```python
from build123d import *

# Parameters (mm, degrees)
BOSS_EXTRUDE1_DEPTH = 12.2
SKETCH2_R           = 1
CUT_EXTRUDE1_DEPTH  = 12.5
SKETCH3_R           = 2.5
BOSS_EXTRUDE2_DEPTH = 4
CUT_EXTRUDE2_DEPTH  = 7.5
SKETCH5_W           = 2.772136711
SKETCH5_H           = 1.05
SKETCH5_W_2         = 2.613565213
SKETCH5_H_2         = 1
CUT_EXTRUDE3_DEPTH  = 7.5


with BuildPart() as part:
    # Sketch1 → Boss-Extrude1 (new body)
    with BuildSketch(Plane.XY):
        Polygon((-5.25, 21), (-5.25, 18.3), (0, 18.3), (0, 0), (22.9, 0), (22.9, 18.3), (28.15, 18.3), (28.15, 21), (22.9, 21), (22.9, 28.5), (0, 28.5), (0, 21), align=None)
    extrude(amount=BOSS_EXTRUDE1_DEPTH)

    # Sketch2 → Cut-Extrude1 (cut)
    with BuildSketch(Plane(origin=(0, 21, 0), x_dir=(1, 0, 0), z_dir=(0, 1, 0))):
        with Locations((-2.55, -6.1)):
            Circle(SKETCH2_R)
        with Locations((25.45, -6.1)):
            Circle(SKETCH2_R)
    extrude(amount=-CUT_EXTRUDE1_DEPTH, mode=Mode.SUBTRACT)

    # Sketch3 → Boss-Extrude2 (add)
    with BuildSketch(Plane(origin=(0, 28.5, 0), x_dir=(1, 0, 0), z_dir=(0, 1, 0))):
        with Locations((6.05, -6.1)):
            Circle(SKETCH3_R)
    extrude(amount=BOSS_EXTRUDE2_DEPTH)

    # Sketch4 → Cut-Extrude2 (cut)
    with BuildSketch(Plane(origin=(0, 28.5, 0), x_dir=(1, 0, 0), z_dir=(0, 1, 0))):
        with BuildLine():
            Line((6.050000045, 0), (0, 0))
            Line((0, 0), (0, -5.320577137))
            ThreePointArc((0, -5.320577137), (2.021630587, -1.519362504), (6.050000045, 0))
        make_face()
        with BuildLine():
            Line((22.9, 0), (6.050000045, 0))
            ThreePointArc((6.050000045, 0), (9.58624096, -1.129587555), (11.812811814, -4.1))
            Line((11.812811814, -4.1), (15.4, -4.1))
            ThreePointArc((15.4, -4.1), (17.4, -6.1), (15.4, -8.1))
            Line((15.4, -8.1), (11.812811814, -8.1))
            ThreePointArc((11.812811814, -8.1), (9.586240956, -11.070412448), (6.050000034, -12.2))
            Line((6.050000034, -12.2), (22.9, -12.2))
            Line((22.9, -12.2), (22.9, 0))
        make_face()
        with BuildLine():
            ThreePointArc((6.050000034, -12.2), (2.021630582, -10.680637492), (0, -6.879422863))
            Line((0, -6.879422863), (0, -12.2))
            Line((0, -12.2), (6.050000034, -12.2))
        make_face()
    extrude(amount=-CUT_EXTRUDE2_DEPTH, mode=Mode.SUBTRACT)

    # Sketch5 → Cut-Extrude3 (cut)
    with BuildSketch(Plane(origin=(0, 21, 0), x_dir=(1, 0, 0), z_dir=(0, 1, 0))):
        with Locations((-3.863931645, -6.125)):
            Rectangle(SKETCH5_W, SKETCH5_H)
        with Locations((26.843217394, -6.1)):
            Rectangle(SKETCH5_W_2, SKETCH5_H_2)
    extrude(amount=-CUT_EXTRUDE3_DEPTH, mode=Mode.SUBTRACT)


solid = part.part
```
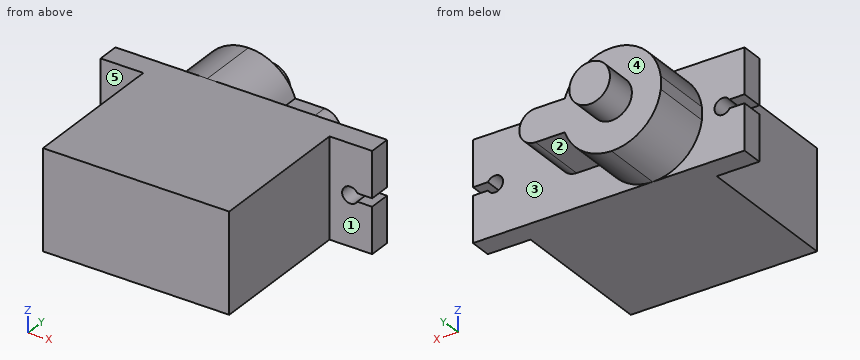
Read the model definition and answer for the solid it produces. Units are mm, in the model's axes. Face numbers are marked on the shaded views. A direction names the side the tool comes from. Coordinates: 2 decimals unless noted, no trailing zeros. Loops run counter-clockwise (first coordinate to the right, second up) from the corner with the lowest first, then second, coordinate; pieces in that order, holes last. Notation, with made-up numbers: (64.25, -18.5) -> (72.25, -18.5) arc R19 ccw to (72.25, 17.5) -> close; hole circle Ø1 at (88.5, 74). An arc over 180 degrees is marked (long way). Return JSON: item names as keys, results as strings.
Item 1: Find section C-C (y = 8). Determine the outline of the cut face in (x, z).
Answers:
{"outline": "(0, 0) -> (22.9, 0) -> (22.9, 12.2) -> (0, 12.2) -> close"}
Item 2: Find the intervals of material crossed by probe 1 along Z at (x, y) = (-2.55, 19.85); probe 2 along Y at (x, z) = (10, 6.25); probe 3 along X at (y, z) = (19.5, 6.1), in increasing order.
Answers:
{"probe 1": "z = 0 to 5.1, 7.1 to 12.2", "probe 2": "y = 0 to 28.5", "probe 3": "x = -1.55 to 24.45"}
Item 3: Find section B-B (z = 6.1). Determine the outline of the cut face in (x, y).
Answers:
{"outline": "(-1.55, 18.3) -> (0, 18.3) -> (0, 0) -> (22.9, 0) -> (22.9, 18.3) -> (24.45, 18.3) -> (24.45, 21) -> (17.4, 21) -> (17.4, 28.5) -> (8.55, 28.5) -> (8.55, 32.5) -> (3.55, 32.5) -> (3.55, 28.5) -> (0, 28.5) -> (0, 21) -> (-1.55, 21) -> close"}
Item 4: For the marked faces 1, 2, 3, 4 and 5, determine the directions among +Z, -Z, +X, -X, +Y, -Y from which every point of the face is accessible in a straight line to the end or side of a thin tool.
Answers:
{"face 1": "+Z, -Z, +X, -Y", "face 2": "-Z, +X, +Y", "face 3": "+X, +Y", "face 4": "+Y", "face 5": "+Z, -Z, -X, -Y"}
Item 5: Find section A-A (x = -2.55). Determine the outline of the cut face in (y, z).
Answers:
{"outline": "(18.3, 0) -> (21, 0) -> (21, 5.1) -> (18.3, 5.1) -> close; (18.3, 7.1) -> (21, 7.1) -> (21, 12.2) -> (18.3, 12.2) -> close"}
Item 6: Flat-ended cylindrical pins translate along their axes: P1, Ø1.8, axis at x = 14.5, y = 25.5, coming from the +Z side; P2, Ø3, axis at x = 24.5, z = 5, coming from the -Y side; P3, Ø1, axis at y = 10, z = 5.5, coming from the +X side. Find the tip coordinate at first contact, or state that the pin passes through.
Answers:
{"P1": "stops at z = 8.1", "P2": "stops at y = 18.3", "P3": "stops at x = 22.9"}
Item 7: Find section D-D (x = 16). Determine the outline of the cut face in (y, z).
Answers:
{"outline": "(0, 0) -> (21, 0) -> (21, 4.19) -> (28.5, 4.19) -> (28.5, 8.01) -> (21, 8.01) -> (21, 12.2) -> (0, 12.2) -> close"}
